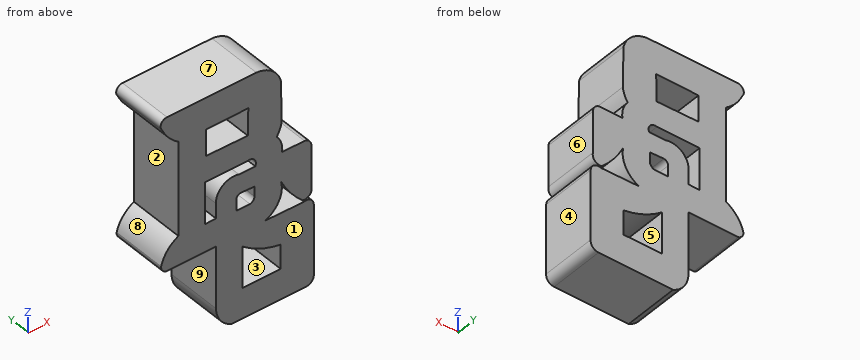
```python
from build123d import *

# Parameters (mm, degrees)
F1_DEPTH = 15
F2_DEPTH = 2.5
F3_DEPTH = 25


with BuildPart() as f1:
    # F0 (on Front) → F1 (new body)
    with BuildSketch(Plane.XZ):
        with BuildLine():
            ThreePointArc((-34.751754, 51.786974), (-31.688129, 46.832693), (-27.364016, 42.92978))
            Line((-27.364016, 42.92978), (-27.364016, 0.631911))
            ThreePointArc((-27.364016, 0.631911), (-32.344059, -3.421449), (-35.177484, -9.18359))
            ThreePointArc((-35.177484, -9.18359), (-34.671706, -11.266714), (-32.907836, -12.4849))
            Line((-32.907836, -12.4849), (-10.331013, -12.4849))
            Line((-10.331013, -12.4849), (-10.331013, -40.363941))
            ThreePointArc((-10.331013, -40.363941), (-8.440878, -46.57815), (-3.410706, -50.687455))
            Line((-3.410706, -50.687455), (30.331215, -50.687455))
            ThreePointArc((30.331215, -50.687455), (33.010256, -49.475316), (33.868331, -46.6628))
            Line((33.868331, -46.6628), (33.868331, -15.41826))
            ThreePointArc((33.868331, -15.41826), (32.369677, -12.53986), (29.152177, -12.116951))
            Line((29.152177, -12.116951), (11.938204, -11.881143))
            ThreePointArc((11.938204, -11.881143), (18.050529, -6.295658), (19.130344, 1.913616))
            ThreePointArc((19.130344, 1.913616), (23.351533, -5.064206), (28.793937, -11.137811))
            ThreePointArc((28.793937, -11.137811), (32.039808, -10.233968), (32.788105, -6.948748))
            Line((32.788105, -6.948748), (32.788105, 11.612454))
            ThreePointArc((32.788105, 11.612454), (31.89459, 13.962579), (29.665431, 15.125466))
            Line((29.665431, 15.125466), (19.534895, 15.125466))
            ThreePointArc((19.534895, 15.125466), (19.187726, 19.388686), (17.125975, 23.13632))
            ThreePointArc((17.125975, 23.13632), (18.607422, 25.946601), (19.366147, 29.031517))
            Line((19.366147, 29.031517), (19.012436, 47.306627))
            ThreePointArc((19.012436, 47.306627), (14.987699, 53.732755), (7.929467, 56.503132))
            Line((7.929467, 56.503132), (-32.511577, 56.503132))
            ThreePointArc((-32.511577, 56.503132), (-35.122158, 54.853038), (-34.751754, 51.786974))
        make_face()
        with BuildLine():
            Line((1.638178, -37.033778), (1.638178, -18.418202))
            ThreePointArc((1.638178, -18.418202), (9.7814, -23.388924), (18.930372, -26.09382))
            Line((18.930372, -26.09382), (18.930372, -37.033778))
            Line((18.930372, -37.033778), (1.638178, -37.033778))
        make_face(mode=Mode.SUBTRACT)
        with BuildLine():
            Line((0.779622, 6.056475), (7.012051, 5.82512))
            Line((7.012051, 5.82512), (7.025873, 1.415433))
            ThreePointArc((7.025873, 1.415433), (6.459904, -0.16527), (5.013869, -1.018453))
            Line((5.013869, -1.018453), (-1.193664, -1.018453))
            Line((-1.193664, -1.018453), (-1.193664, 3.909603))
            ThreePointArc((-1.193664, 3.909603), (-0.625401, 5.367591), (0.779622, 6.056475))
        make_face(mode=Mode.SUBTRACT)
        with BuildLine():
            Line((-15.418217, 0), (-15.418217, 18.833645))
            Line((-15.418217, 18.833645), (3.903346, 18.833645))
            ThreePointArc((3.903346, 18.833645), (6.97837, 17.914546), (7.416358, 14.735131))
            Line((7.416358, 14.735131), (0, 14.735131))
            ThreePointArc((0, 14.735131), (-7.187256, 13.466433), (-10.416982, 6.921578))
            Line((-10.416982, 6.921578), (-10.345434, 0.052841))
            Line((-10.345434, 0.052841), (-15.418217, 0))
        make_face(mode=Mode.SUBTRACT)
        Polygon((-14.898672, 30.383811), (-14.898672, 42.196874), (4.256723, 42.367905), (4.034158, 30.126804), align=None, mode=Mode.SUBTRACT)
    extrude(amount=F1_DEPTH)

    # F0 (on Front) → F2 (cut, symmetric)
    with BuildSketch(Plane.XZ):
        with BuildLine():
            ThreePointArc((-34.751754, 51.786974), (-31.688129, 46.832693), (-27.364016, 42.92978))
            Line((-27.364016, 42.92978), (-27.364016, 0.631911))
            ThreePointArc((-27.364016, 0.631911), (-32.344059, -3.421449), (-35.177484, -9.18359))
            ThreePointArc((-35.177484, -9.18359), (-34.671706, -11.266714), (-32.907836, -12.4849))
            Line((-32.907836, -12.4849), (-10.331013, -12.4849))
            Line((-10.331013, -12.4849), (-10.331013, -40.363941))
            ThreePointArc((-10.331013, -40.363941), (-8.440878, -46.57815), (-3.410706, -50.687455))
            Line((-3.410706, -50.687455), (30.331215, -50.687455))
            ThreePointArc((30.331215, -50.687455), (33.010256, -49.475316), (33.868331, -46.6628))
            Line((33.868331, -46.6628), (33.868331, -15.41826))
            ThreePointArc((33.868331, -15.41826), (32.369677, -12.53986), (29.152177, -12.116951))
            Line((29.152177, -12.116951), (11.938204, -11.881143))
            ThreePointArc((11.938204, -11.881143), (18.050529, -6.295658), (19.130344, 1.913616))
            ThreePointArc((19.130344, 1.913616), (23.351533, -5.064206), (28.793937, -11.137811))
            ThreePointArc((28.793937, -11.137811), (32.039808, -10.233968), (32.788105, -6.948748))
            Line((32.788105, -6.948748), (32.788105, 11.612454))
            ThreePointArc((32.788105, 11.612454), (31.89459, 13.962579), (29.665431, 15.125466))
            Line((29.665431, 15.125466), (19.534895, 15.125466))
            ThreePointArc((19.534895, 15.125466), (19.187726, 19.388686), (17.125975, 23.13632))
            ThreePointArc((17.125975, 23.13632), (18.607422, 25.946601), (19.366147, 29.031517))
            Line((19.366147, 29.031517), (19.012436, 47.306627))
            ThreePointArc((19.012436, 47.306627), (14.987699, 53.732755), (7.929467, 56.503132))
            Line((7.929467, 56.503132), (-32.511577, 56.503132))
            ThreePointArc((-32.511577, 56.503132), (-35.122158, 54.853038), (-34.751754, 51.786974))
        make_face()
        with BuildLine():
            Line((1.638178, -37.033778), (1.638178, -18.418202))
            ThreePointArc((1.638178, -18.418202), (9.7814, -23.388924), (18.930372, -26.09382))
            Line((18.930372, -26.09382), (18.930372, -37.033778))
            Line((18.930372, -37.033778), (1.638178, -37.033778))
        make_face(mode=Mode.SUBTRACT)
        with BuildLine():
            Line((0.779622, 6.056475), (7.012051, 5.82512))
            Line((7.012051, 5.82512), (7.025873, 1.415433))
            ThreePointArc((7.025873, 1.415433), (6.459904, -0.16527), (5.013869, -1.018453))
            Line((5.013869, -1.018453), (-1.193664, -1.018453))
            Line((-1.193664, -1.018453), (-1.193664, 3.909603))
            ThreePointArc((-1.193664, 3.909603), (-0.625401, 5.367591), (0.779622, 6.056475))
        make_face(mode=Mode.SUBTRACT)
        with BuildLine():
            Line((-15.418217, 0), (-15.418217, 18.833645))
            Line((-15.418217, 18.833645), (3.903346, 18.833645))
            ThreePointArc((3.903346, 18.833645), (6.97837, 17.914546), (7.416358, 14.735131))
            Line((7.416358, 14.735131), (0, 14.735131))
            ThreePointArc((0, 14.735131), (-7.187256, 13.466433), (-10.416982, 6.921578))
            Line((-10.416982, 6.921578), (-10.345434, 0.052841))
            Line((-10.345434, 0.052841), (-15.418217, 0))
        make_face(mode=Mode.SUBTRACT)
        Polygon((-14.898672, 30.383811), (-14.898672, 42.196874), (4.256723, 42.367905), (4.034158, 30.126804), align=None, mode=Mode.SUBTRACT)
    extrude(amount=F2_DEPTH, both=True, mode=Mode.SUBTRACT)

    # F0 (on Front) → F3 (join)
    with BuildSketch(Plane.XZ):
        with BuildLine():
            ThreePointArc((-34.751754, 51.786974), (-31.688129, 46.832693), (-27.364016, 42.92978))
            Line((-27.364016, 42.92978), (-27.364016, 0.631911))
            ThreePointArc((-27.364016, 0.631911), (-32.344059, -3.421449), (-35.177484, -9.18359))
            ThreePointArc((-35.177484, -9.18359), (-34.671706, -11.266714), (-32.907836, -12.4849))
            Line((-32.907836, -12.4849), (-10.331013, -12.4849))
            Line((-10.331013, -12.4849), (-10.331013, -40.363941))
            ThreePointArc((-10.331013, -40.363941), (-8.440878, -46.57815), (-3.410706, -50.687455))
            Line((-3.410706, -50.687455), (30.331215, -50.687455))
            ThreePointArc((30.331215, -50.687455), (33.010256, -49.475316), (33.868331, -46.6628))
            Line((33.868331, -46.6628), (33.868331, -15.41826))
            ThreePointArc((33.868331, -15.41826), (32.369677, -12.53986), (29.152177, -12.116951))
            Line((29.152177, -12.116951), (11.938204, -11.881143))
            ThreePointArc((11.938204, -11.881143), (18.050529, -6.295658), (19.130344, 1.913616))
            ThreePointArc((19.130344, 1.913616), (23.351533, -5.064206), (28.793937, -11.137811))
            ThreePointArc((28.793937, -11.137811), (32.039808, -10.233968), (32.788105, -6.948748))
            Line((32.788105, -6.948748), (32.788105, 11.612454))
            ThreePointArc((32.788105, 11.612454), (31.89459, 13.962579), (29.665431, 15.125466))
            Line((29.665431, 15.125466), (19.534895, 15.125466))
            ThreePointArc((19.534895, 15.125466), (19.187726, 19.388686), (17.125975, 23.13632))
            ThreePointArc((17.125975, 23.13632), (18.607422, 25.946601), (19.366147, 29.031517))
            Line((19.366147, 29.031517), (19.012436, 47.306627))
            ThreePointArc((19.012436, 47.306627), (14.987699, 53.732755), (7.929467, 56.503132))
            Line((7.929467, 56.503132), (-32.511577, 56.503132))
            ThreePointArc((-32.511577, 56.503132), (-35.122158, 54.853038), (-34.751754, 51.786974))
        make_face()
        with BuildLine():
            Line((1.638178, -37.033778), (1.638178, -18.418202))
            ThreePointArc((1.638178, -18.418202), (9.7814, -23.388924), (18.930372, -26.09382))
            Line((18.930372, -26.09382), (18.930372, -37.033778))
            Line((18.930372, -37.033778), (1.638178, -37.033778))
        make_face(mode=Mode.SUBTRACT)
        with BuildLine():
            Line((0.779622, 6.056475), (7.012051, 5.82512))
            Line((7.012051, 5.82512), (7.025873, 1.415433))
            ThreePointArc((7.025873, 1.415433), (6.459904, -0.16527), (5.013869, -1.018453))
            Line((5.013869, -1.018453), (-1.193664, -1.018453))
            Line((-1.193664, -1.018453), (-1.193664, 3.909603))
            ThreePointArc((-1.193664, 3.909603), (-0.625401, 5.367591), (0.779622, 6.056475))
        make_face(mode=Mode.SUBTRACT)
        with BuildLine():
            Line((-15.418217, 0), (-15.418217, 18.833645))
            Line((-15.418217, 18.833645), (3.903346, 18.833645))
            ThreePointArc((3.903346, 18.833645), (6.97837, 17.914546), (7.416358, 14.735131))
            Line((7.416358, 14.735131), (0, 14.735131))
            ThreePointArc((0, 14.735131), (-7.187256, 13.466433), (-10.416982, 6.921578))
            Line((-10.416982, 6.921578), (-10.345434, 0.052841))
            Line((-10.345434, 0.052841), (-15.418217, 0))
        make_face(mode=Mode.SUBTRACT)
        Polygon((-14.898672, 30.383811), (-14.898672, 42.196874), (4.256723, 42.367905), (4.034158, 30.126804), align=None, mode=Mode.SUBTRACT)
    extrude(amount=F3_DEPTH)


solid = f1.part
```
Work out the finished part from the listing and answer in its coordinate system (mm). Face numbers are marked on the shaded views. A direction names the side the tool comes from. Coordinates: 2 decimals unless noted, no trailing zeros. Write each loop counter-clockwise with the first axis right and the second up, starting at its lowest first coordinate (ties: lowest second). Pieces come first, ordered by that corner, then holes.
Q1. Each of these flat-tipped pins is pushed along its axis until it touches: pin 1 Ø11.5 at (x, y) = (-23, -16.5) entering from -Z; pin 2 Ø3 at (y, z) = (-13, 43) entering from -X; pin 3 Ø5 at (y, z) = (-21, 40) entering from -X. Where does it stop, or does it pass through?
Q2. Which of the six approach directions +Z, -Z, +X, -X, +Y, -Y give full straight-line access (tool end or side, diameter ignored) to the marked faces 5, 6, 7, 8 and 9?
Q3. A cutting plane is placed at D-D, the plane x = -20. Give the vertices of the cut face in (y, z), then the cut area to 3 significant figures.
Q4. Determine the mould class of the marked faces 1, 2, 3 and 4 for opening direction X: released by +X, released by -X, zero draft, split by the parting line, or undercut.
Q5. A cutting plane is placed at C-C, the plane y = -7.25. State how many separate pieces and enclosed holes the cut face has, then the cut area to 3 significant figures.
Q6. A cutting plane is placed at A-A, the plane z = -33. Give the vertices of the cut face in (x, y).
Q7. A cutting plane is placed at B-B, the plane x = -29. Give the vertices of the cut face in (y, z).
Q8. Find the intervals of material crossed by line 1 (Z direction, x = 6, y = -5.5); line 2 (Z direction, x = -7, y = -18.25); line 3 (X direction, y = -4.25, z = 0.5), in increasing order.
Findings below:
1. pin 1: stops at z = -12.48
1. pin 2: stops at x = -29.41
1. pin 3: stops at x = -27.36
2. face 5: +Y, -Y
2. face 6: +Z, +X, +Y, -Y
2. face 7: +Z, +X, -X, +Y, -Y
2. face 8: -X, +Y, -Y
2. face 9: -Z, -X, +Y, -Y
3. outline: (-25, -12.48) - (0, -12.48) - (0, 56.5) - (-25, 56.5) - close
3. area: 1,720 mm2
4. face 1: zero draft
4. face 2: released by -X
4. face 3: undercut
4. face 4: released by +X
5. separate pieces: 1
5. enclosed holes: 4
5. area: 4,570 mm2
6. outline: (-10.33, -25) - (1.64, -25) - (1.64, 0) - (-10.33, 0) - close; (18.93, -25) - (33.87, -25) - (33.87, 0) - (18.93, 0) - close
7. outline: (-25, -12.48) - (0, -12.48) - (0, -0.33) - (-25, -0.33) - close; (-25, 44.15) - (0, 44.15) - (0, 56.5) - (-25, 56.5) - close
8. line 1: z = -50.69 to -37.03, -21.44 to -0.6, 5.86 to 14.74, 18.66 to 56.5
8. line 2: z = -48.32 to 13.6, 18.83 to 30.28, 42.27 to 56.5
8. line 3: x = -27.62 to -15.42, -10.35 to -1.19, 6.85 to 19.36, 19.85 to 32.79
